Autodesk Inventor part; units mm, degrees
ref_plane "YZ Plane" through (0, 0, 0) normal (1, 0, 0) x (0, 1, 0)
ref_plane "XZ Plane" through (0, 0, 0) normal (0, 1, 0) x (-1, 0, 0)
ref_plane "XY Plane" through (0, 0, 0) normal (0, 0, 1) x (1, 0, 0)
sketch "Esquisse3" plane through (0, 0, 0) normal (0, 1, 0) x (-1, 0, 0)
  line L0 (-6.5, 6.5) -> (6.5, 6.5) construction
  line L1 (6.5, 6.5) -> (6.5, -6.5) construction
  line L2 (6.5, -6.5) -> (-6.5, -6.5) construction
  line L3 (-6.5, -6.5) -> (-6.5, 6.5) construction
  line L4 (-6.5, 6.5) -> (6.5, -6.5) construction
  line L5 (6.5, 6.5) -> (-6.5, -6.5) construction
  line L6 (-11.5, 11.5) -> (11.5, 11.5) construction
  line L7 (11.5, 11.5) -> (11.5, -11.5) construction
  line L8 (11.5, -11.5) -> (-11.5, -11.5) construction
  line L9 (-11.5, -11.5) -> (-11.5, 11.5) construction
  line L10 (-11.5, 11.5) -> (11.5, -11.5) construction
  line L11 (11.5, 11.5) -> (-11.5, -11.5) construction
  line L12 (-6.5, 6.5) -> (-11.5, 6.5) construction
  line L13 (-11.5, 6.5) -> (-11.5, 11.5) construction
  line L14 (-11.5, 11.5) -> (-6.5, 11.5) construction
  line L15 (-6.5, 11.5) -> (-6.5, 6.5) construction
  line L16 (-6.5, -6.5) -> (-11.5, -6.5) construction
  line L17 (-11.5, -6.5) -> (-11.5, -11.5) construction
  line L18 (-11.5, -11.5) -> (-6.5, -11.5) construction
  line L19 (-6.5, -11.5) -> (-6.5, -6.5) construction
  line L20 (6.5, -6.5) -> (11.5, -6.5) construction
  line L21 (11.5, -6.5) -> (11.5, -11.5) construction
  line L22 (11.5, -11.5) -> (6.5, -11.5) construction
  line L23 (6.5, -11.5) -> (6.5, -6.5) construction
  line L24 (11.5, 11.5) -> (6.5, 11.5) construction
  line L25 (6.5, 11.5) -> (6.5, 6.5) construction
  line L26 (6.5, 6.5) -> (11.5, 6.5) construction
  line L27 (11.5, 6.5) -> (11.5, 11.5) construction
  circle A0 centre (9, 9) radius 2.5
  circle A1 centre (9, -9) radius 2.5
  circle A2 centre (-9, -9) radius 2.5
  circle A3 centre (-9, 9) radius 2.5
  circle A4 centre (0, 0) radius 17.5
  circle A5 centre (0, 0) radius 8.5
  dimension "d1" = 13
  dimension "d2" = 13
  dimension "d3" = 5
  dimension "d4" = 35
  dimension "d9" = 9
extrude "Extrusion1" add sketch "Esquisse3" along normal blind 2
sketch "Esquisse4" plane through (0, 2, 0) normal (0, 1, 0) x (1, 0, 0)
  circle A0 centre (-9, 9) radius 3.5
  circle A1 centre (-9, 9) radius 2.5
  circle A2 centre (9, 9) radius 3.5
  circle A3 centre (9, -9) radius 3.5
  circle A4 centre (-9, -9) radius 3.5
  circle A5 centre (9, 9) radius 2.5
  circle A6 centre (9, -9) radius 2.5
  circle A7 centre (-9, -9) radius 2.5
  circle A8 centre (0, 0) radius 17.5
  circle A9 centre (0, 0) radius 8.544
  circle A10 centre (9, 9) radius 2.5
  circle A11 centre (9, 9) radius 2.5
  circle A12 centre (9, -9) radius 2.5
  circle A13 centre (-9, -9) radius 2.5
  dimension "d10" = 7
  dimension "d11" = 7
  dimension "d12" = 7
  dimension "d13" = 7
extrude "Extrusion2" add sketch "Esquisse4" along normal blind 2 contours A0 | A2 | A3 | A4 | A8
chamfer "Chanfrein1" distance 1 distance2 2 1 edges at (-11.5, 4, -9) measured on face at (3.3085, 4, 12.0053)
chamfer "Chanfrein2" distance 1 distance2 2 1 edges at (6.5, 4, -9) measured on face at (3.3085, 4, 12.0053)
chamfer "Chanfrein3" distance 1 distance2 2 1 edges at (-11.5, 4, 9) measured on face at (3.3085, 4, 12.0053)
chamfer "Chanfrein4" distance 1 distance2 2 1 edges at (6.5, 4, 9) measured on face at (3.3085, 4, 12.0053)
properties part number "Pièce_moteur_maintient_test_2"
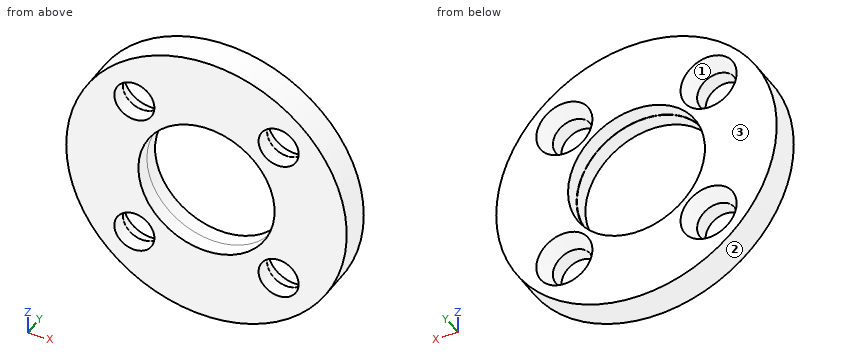
Geometry: final body of the model. Coordinates: model frame, mm. Face numbers are marked on the shaded views. Round coordinates to 2 decimals unless told otherwise and drop trailing zeros. Loops run counter-clockwise (first coordinate to the right, second up) from the corner with the lowest first, then second, coordinate; pieces in that order, holes last. Notation, with made-up numbers: (54.25, 56) -> (62.25, 56) arc R26 ccw to (62.25, 89) -> close; hole circle Ø4 at (11, 89.25). An arc over 180 degrees is marked (long way). Use one line per item in the form item = value. Start each with the question number.
1) Section B-B on y = 3.4. Output: boundary loops of the cut face in (x, z), then the cut area to 3 significant figures.
2) Section A-A on z = -4. Output: boundary loops of the cut face in (x, y).
3) Line query: L1, parallel to Z at x = 0, y = 0.8; L2, parallel to X at y = 2.3, z = 7; L3, parallel to Z at x = -9, y = 0.5. Output: solid intervals per line, ascending.
4) Draft query along Z for the marked faces 1, 2 and 3. Return one class per face: released by +Z, released by -Z, zero draft, split by the parting line, or undercut.
5) Section D-D on z = -15. Output: boundary loops of the cut face in (x, y).
6) First-contact query: P1, Ø2, axis at x = -2.5, y = 1.5, coming from the +Z side; P2, Ø5, axis at x = 9, z = -9.5, coming from the +Y side; P3, Ø1.5, axis at y = 1.5, z = -6, coming from the -X side. Flat tips, straight axial feed; report the tip coordinate or a pass-through.
Response:
q1.outline = circle Ø35 at (0, 0); hole circle Ø6.4 at (-9, -9); hole circle Ø6.4 at (-9, 9); hole circle Ø17.09 at (0, 0); hole circle Ø6.4 at (9, -9); hole circle Ø6.4 at (9, 9)
q1.area = 604 mm^2
q2.outline = (-17.04, 0) -> (-7.5, 0) -> (-7.5, 2) -> (-7.55, 2) -> (-7.55, 4) -> (-17.04, 4) -> close; (7.5, 0) -> (17.04, 0) -> (17.04, 4) -> (7.55, 4) -> (7.55, 2) -> (7.5, 2) -> close
q3.L1 = -17.5 to -8.5, 8.5 to 17.5
q3.L2 = -16.04 to -10.74, -7.26 to -4.9, 4.9 to 7.26, 10.74 to 16.04
q3.L3 = -15.01 to -11.5, -6.5 to 6.5, 11.5 to 15.01
q4.face_1 = undercut
q4.face_2 = split by the parting line
q4.face_3 = zero draft
q5.outline = (-9.01, 0) -> (9.01, 0) -> (9.01, 4) -> (-9.01, 4) -> close
q6.P1 = 17.44
q6.P2 = 3
q6.P3 = -16.69
